from build123d import *

# Parameters (mm, degrees)
SKIZZE1_R                       = 17.5
AUFSATZ_LINEAR_AUSTRAGEN1_DEPTH = 3
SKIZZE2_R                       = 1
SCHNITT_LINEAR_AUSTRAGEN1_DEPTH = 25.929901725


with BuildPart() as part:
    # Skizze1 → Aufsatz-Linear austragen1 (new body)
    with BuildSketch(Plane(origin=(0, 0, 0), x_dir=(1, 0, 0), z_dir=(0, 1, 0))):
        with Locations(Location((0, 0, 0), (0, 0, 270))):
            Circle(SKIZZE1_R)
    extrude(amount=AUFSATZ_LINEAR_AUSTRAGEN1_DEPTH)

    # Skizze2 → Schnitt-Linear austragen1 (cut, through all)
    with BuildSketch(Plane(origin=(0, 3, 0), x_dir=(1, 0, 0), z_dir=(0, 1, 0))):
        with Locations(Location((-7.5, 0, 0), (0, 0, 270))):
            Circle(SKIZZE2_R)
        with Locations(Location((7.5, 0, 0), (0, 0, 270))):
            Circle(SKIZZE2_R)
        with BuildLine():
            Line((-1.658312395, 2.5), (1.658312395, 2.5))
            ThreePointArc((1.658312395, 2.5), (0, -3), (-1.658312395, 2.5))
        make_face()
    extrude(amount=-SCHNITT_LINEAR_AUSTRAGEN1_DEPTH, mode=Mode.SUBTRACT)


solid = part.part
Source: CAD feature listing. Evaluate the final solid. Frame: model axes, mm. A direction names the side the tool comes from. Coordinates: 2 decimals unless noted, no trailing zeros. Loops run counter-clockwise (first coordinate to the right, second up) from the corner with the lowest first, then second, coordinate; pieces in that order, holes last. Notation, with made-up numbers: (19, 89) - (35, 89) arc R18 ccw to (35, 96) - close; hole circle Ø4 at (-4, -2). An arc over 180 degrees is marked (long way). One line per question, with ' | ' between items.
1) First-contact query: P1, Ø1, axis at y = 1.5, z = -6, coming from the -X side; P2, Ø1.2, axis at x = 7.5, z = 0, coming from the -Y side; P3, Ø1, axis at x = 9.5, y = 1.5, coming from the +Z side. Flat tips, straight axial feed; report the tip coordinate or a pass-through.
Report:
P1: stops at x = -16.61 | P2: passes through | P3: stops at z = 15.01
2) Section B-B, the plane z = 0. Return loops of the section in (x, y), then the cut area to 3 significant figures.
Report:
outline: (-17.5, 0) - (-8.5, 0) - (-8.5, 3) - (-17.5, 3) - close; (-6.5, 0) - (-3, 0) - (-3, 3) - (-6.5, 3) - close; (3, 0) - (6.5, 0) - (6.5, 3) - (3, 3) - close; (8.5, 0) - (17.5, 0) - (17.5, 3) - (8.5, 3) - close | area: 75.0 mm²
3) Set-up query: faces 1 (the face through (0, 2, -2.5)), 2 (the face through (-4, 3, 0)). Return all of +Z, -Z, +X, -X, +Y, -Y with unobstructed straight access to the full face (end or side cutting, diameter ignored); none if empty.
Report:
face 1: +Y, -Y | face 2: +Z, -Z, +X, -X, +Y
4) Pull-direction query (Z, two-part tool) for faces 3 (the face through (-4, 0, 0)), 4 (the face through (-10.648, 1.479, -13.887)), 5 (the face through (8.49, 1.52, -0.13)); classes: released by +Z, released by -Z, zero draft, split by the parting line, or undercut.
Report:
face 3: zero draft | face 4: split by the parting line | face 5: undercut
5) Section C-C, the plane y = 1.25. Return loops of the section in (x, z), then the cut area to 3 significant figures.
Report:
outline: circle Ø35 at (0, 0); hole circle Ø2 at (-7.5, 0); hole (-1.66, -2.5) - (1.66, -2.5) arc R3 ccw (long way) to start; hole circle Ø2 at (7.5, 0) | area: 929 mm²
6) Section A-A, the plane x = 0. Return loops of the section in (y, z), then the cut area to 3 significant figures.
Report:
outline: (0, -17.5) - (3, -17.5) - (3, -2.5) - (0, -2.5) - close; (0, 3) - (3, 3) - (3, 17.5) - (0, 17.5) - close | area: 88.5 mm²
7) Section D-D, the plane x = -7.5. Return loops of the section in (y, z), then the cut area to 3 significant figures.
Report:
outline: (0, -15.81) - (3, -15.81) - (3, -1) - (0, -1) - close; (0, 1) - (3, 1) - (3, 15.81) - (0, 15.81) - close | area: 88.9 mm²
8) Line query: line 1 along X through (y, z) = (1.35, 0); line 2 along Z through (x, y) = (-2.5, 1.05); line 3 along Z through (x, y) = (1, 2.3). Output: solid intervals per line, ascending.
Report:
line 1: x = -17.5 to -8.5, -6.5 to -3, 3 to 6.5, 8.5 to 17.5 | line 2: z = -17.32 to -1.66, 1.66 to 17.32 | line 3: z = -17.47 to -2.5, 2.83 to 17.47
